Autodesk Inventor part; units mm, degrees
ref_plane "YZ Plane" through (0, 0, 0) normal (1, 0, 0) x (0, 1, 0)
ref_plane "XZ Plane" through (0, 0, 0) normal (0, 1, 0) x (-1, 0, 0)
ref_plane "XY Plane" through (0, 0, 0) normal (0, 0, 1) x (1, 0, 0)
sketch "Sketch4" plane through (0, 0, 0) normal (0, 0, 1) x (1, 0, 0)
  arc A0 (-0.0698, 6.3496) -> (6.1152, -1.7109) centre (0, 0) ccw
  arc A1 (-0.9946, 7.5548) -> (7.04, -2.916) centre (0, 0) ccw
  line L0 (0, 0) -> (0, 7.9375) construction
  line L1 (-0.0698, 6.3496) -> (6.1152, -1.7109) construction
  line L2 (-0.0698, 6.3496) -> (-0.9946, 7.5548)
  line L3 (6.1152, -1.7109) -> (7.04, -2.916)
  circle A2 centre (0, 0) radius 6.35
  dimension "d10" = 12.7
  dimension "d11" = 1.27
  dimension "d12" = 37.5
  dimension "d13" = 10.16
extrude "Extrusion3" add sketch "Sketch4" along normal mid plane 38.1 contours A0 L3 A1 L2
sketch "Sketch5" plane through (0, 0, 0) normal (0, 0, 1) x (1, 0, 0)
  arc A0 (-0.9946, 7.5548) -> (7.04, -2.916) centre (0, 0) ccw
  line L0 (-7.62, 0) -> (-7.62, -29.21)
  line L1 (-7.62, -29.21) -> (0, -29.21)
  line L2 (0, -29.21) -> (0, -7.62)
  circle A1 centre (0, 0) radius 7.9375
  dimension "d16" = 21.59
extrude "Extrusion4" add sketch "Sketch5" along normal mid plane 38.1 contours A0 L2 A1 L0 | A1 L2 L1 L0 picked at (-7.3048, -2.4081)
sketch "Sketch6" plane through (0, -29.21, 19.05) normal (1, 0, 0) x (0, 0, -1)
  line L0 (0, 21.59) -> (38.1, 21.59)
  line L1 (38.1, 21.59) -> (38.1, 0)
  line L2 (0, 0) -> (38.1, 0)
  line L3 (0, 0) -> (0, 21.59)
  line L4 (19.05, 0) -> (19.05, 21.59) construction
  point P0 (19.05, 29.21)
  point P1 (19.05, 5.08)
  dimension "d30" = 5.08
  dimension "d31" = 0
hole "Hole1" at (0, -24.13, 0) direction (-1, 0, 0) diameter 3.5052 end through all countersink diameter 7.112 countersink angle 82
sketch "Sketch10" plane through (-7.62, -29.21, 19.05) normal (0, -1, 0) x (1, 0, 0)
  line L0 (0, -38.1) -> (0, 0)
  line L1 (7.62, -38.1) -> (0, -38.1)
  line L2 (7.62, 0) -> (7.62, -38.1)
  line L3 (0, 0) -> (7.62, 0)
  line L4 (3.81, -38.1) -> (3.81, 0) construction
  spline S0 degree 2 poles (2.8014, -21.2421) (3.1307, -21.2421) (3.7235, -21.4768) (3.9294, -21.6867) knots 0 0 0 1 2 2 2
  spline S1 degree 2 poles (3.9294, -21.6867) (4.1887, -21.9502) (4.4563, -22.6624) (4.4563, -23.2058) knots 0 0 0 1 2 2 2
  line L5 (4.4563, -23.2058) -> (4.4563, -23.778)
  line L6 (4.4563, -23.778) -> (6.35, -23.778)
  line L7 (6.35, -23.778) -> (6.35, -24.4532)
  line L8 (6.35, -24.4532) -> (1.27, -24.4532)
  line L9 (1.27, -24.4532) -> (1.27, -23.177)
  spline S2 degree 2 poles (1.27, -23.177) (1.27, -22.7241) (1.4182, -22.0902) (1.587, -21.8473) knots 0 0 0 1 2 2 2
  spline S3 degree 2 poles (1.587, -21.8473) (1.7805, -21.5632) (2.3774, -21.2421) (2.8014, -21.2421) knots 0 0 0 1 2 2 2
  spline S4 degree 2 poles (2.822, -21.9461) (2.5585, -21.9461) (2.1716, -22.1272) (2.0481, -22.3125) knots 0 0 0 1 2 2 2
  spline S5 degree 2 poles (2.0481, -22.3125) (1.941, -22.473) (1.8546, -22.9012) (1.8546, -23.2182) knots 0 0 0 1 2 2 2
  line L10 (1.8546, -23.2182) -> (1.8546, -23.778)
  line L11 (1.8546, -23.778) -> (3.88, -23.778)
  line L12 (3.88, -23.778) -> (3.88, -23.317)
  spline S6 degree 2 poles (3.88, -23.317) (3.88, -22.9053) (3.7482, -22.3989) (3.5753, -22.2343) knots 0 0 0 1 2 2 2
  spline S7 degree 2 poles (3.5753, -22.2343) (3.423, -22.0819) (3.0649, -21.9461) (2.822, -21.9461) knots 0 0 0 1 2 2 2
  line L13 (1.27, -16.9155) -> (6.35, -18.6651)
  line L14 (6.35, -18.6651) -> (6.35, -19.3937)
  line L15 (6.35, -19.3937) -> (1.27, -21.1433)
  line L16 (1.27, -21.1433) -> (1.27, -20.4188)
  line L17 (1.27, -20.4188) -> (5.4896, -19.0109)
  line L18 (5.4896, -19.0109) -> (1.27, -17.603)
  line L19 (1.27, -17.603) -> (1.27, -16.9155)
  line L20 (6.35, -13.3834) -> (6.35, -16.5162)
  line L21 (6.35, -16.5162) -> (5.6296, -16.5162)
  spline S8 degree 2 poles (5.6296, -16.5162) (5.3126, -16.1786) (4.7239, -15.5776) (4.4069, -15.2894) knots 0 0 0 1 2 2 2
  spline S9 degree 2 poles (4.4069, -15.2894) (3.7688, -14.7089) (3.0031, -14.2849) (2.5956, -14.2849) knots 0 0 0 1 2 2 2
  spline S10 degree 2 poles (2.5956, -14.2849) (2.3815, -14.2849) (2.0604, -14.4167) (1.9575, -14.536) knots 0 0 0 1 2 2 2
  spline S11 degree 2 poles (1.9575, -14.536) (1.8546, -14.6554) (1.7517, -14.9683) (1.7517, -15.1577) knots 0 0 0 1 2 2 2
  spline S12 degree 2 poles (1.7517, -15.1577) (1.7517, -15.3388) (1.8422, -15.7093) (1.9122, -15.8781) knots 0 0 0 1 2 2 2
  spline S13 degree 2 poles (1.9122, -15.8781) (1.9698, -16.0222) (2.1345, -16.2898) (2.1921, -16.3721) knots 0 0 0 1 2 2 2
  line L22 (2.1921, -16.3721) -> (2.1921, -16.4091)
  line L23 (2.1921, -16.4091) -> (1.4676, -16.4091)
  spline S14 degree 2 poles (1.4676, -16.4091) (1.3647, -16.1992) (1.163, -15.4458) (1.163, -15.1083) knots 0 0 0 1 2 2 2
  spline S15 degree 2 poles (1.163, -15.1083) (1.163, -14.3961) (1.9163, -13.5933) (2.5585, -13.5933) knots 0 0 0 1 2 2 2
  spline S16 degree 2 poles (2.5585, -13.5933) (2.859, -13.5933) (3.3613, -13.7333) (3.5753, -13.8568) knots 0 0 0 1 2 2 2
  spline S17 degree 2 poles (3.5753, -13.8568) (3.7976, -13.9803) (4.234, -14.3384) (4.444, -14.536) knots 0 0 0 1 2 2 2
  spline S18 degree 2 poles (4.444, -14.536) (4.7939, -14.8571) (5.5431, -15.6434) (5.7613, -15.8781) knots 0 0 0 1 2 2 2
  line L24 (5.7613, -15.8781) -> (5.7613, -13.3834)
  line L25 (5.7613, -13.3834) -> (6.35, -13.3834)
  point P0 (7.62, -19.05)
extrude "Text" cut sketch "Sketch10" against normal blind 1.143 contours S0 S1 L5 L6 L7 L8 L9 S2 S3 | L13 L14 L15 L16 L17 L18 L19 | L20 L21 S8 S9 S10 S11 S12 S13 L22 L23 S14 S15 S16 S17 S18 L24 L25
equation "\"d10\" = shadeDiameter"
equation "\"d11\" = shadeHolderWallThickness"
equation "\"d13\" = openingForShade"
equation "\"d14\" = partWidth"
equation "\"d16\" = flatBelowShade"
equation "\"d17\" = partWidth"
equation "\"d28\" = textDepth"
equation "\"shadeDiameter\" = 12.7"
equation "\"partWidth\" = 38.1"
equation "\"backThickness\" = 1.905"
equation "\"backHeight\" = 25.4"
equation "\"cutTiltAngle\" = 52.5deg"
equation "\"flatBelowShade\" = 21.59"
equation "\"shadeHolderWallThickness\" = 1.27"
equation "\"openingForShade\" = 10.16"
equation "\"textDepth\" = 1.143"
equation "\"holeHeightAboveBottom\" = 5.08"
properties part number "shadeHolderSideWindow"
Check sheet for the modelled part. Datum: model origin and axes. Units: mm. A direction names the side the tool comes from. Give positions to 0.01 mm unless a question says otherwise; leave off trailing zeros. Loops run counter-clockwise (first coordinate to the right, second up) from the corner with the lowest first, then second, coordinate; pieces in that order, holes last. Notation, with made-up numbers: (32, 19.25) - (37, 19.25) arc R11 cw to (37, 31.25) - close; hole circle Ø8 at (-16, 24.5). An arc over 180 degrees is marked (long way). One line per question, with ' | ' between items. Start each with the question number.
1. Material ranges on line 1 along Y through (x, z) = (-4.5, 1); line 2 along Y through (x, z) = (-5.3, 0); line 3 along X through (y, z) = (-20, 8.5), recorded low to high. Write a range as [from, to].
2. Gauge pin test, flat ends, axial feed: pin 1 Ø0.9 at (y, z) = (-28.5, 4.5) entering from +X; pin 2 Ø4.5 at (y, z) = (-24.13, 0) entering from +X; pin 3 Ø1 at (x, y) = (2.5, -3.5) entering from -Z. Record the tip position at first contact, or that the pin passes through.
3. Cross-section at C-C, the plane x = 5. Enter the section's corners in (y, z), plus the area to 3 significant figures.
4. Cross-section at D-D, the plane y = -17.5. Enter the section's corners in (x, z), plus the area to 3 significant figures.
5. Set-up check for faces 4 (the flat face through (-5, -29.21, -4)), 5 (the flat face through (0, -19, 0)), 6 (the flat face through (-5, -29, -4.728)): record each of +Z, -Z, +X, -X, +Y, -Y from which the full face is reachable in a straight line by a thin tool's end or side.
6. Cross-section at A-A, the plane y = -24.13. Enter the section's corners in (x, z), plus the area to 3 significant figures.
7. Cross-section at B-B, the plane z = 11. Enter the section's corners in (x, y).
8. Draft check along Z on faces 1 (the flat face through (-4, -15, 19.05)), 2 (the flat face through (-4, -29.21, 0)), 3 (the flat face through (-3.846, -28.647, 1.272)). Enter one of: released by +Z, released by -Z, zero draft, split by the parting line, or undercut.
Check result:
1) line 1: y = [-28.07, -25.57], [-22.69, -4.48], [4.48, 6.15] | line 2: y = [-29.21, -25.88], [-22.38, -3.5], [3.5, 5.47] | line 3: x = [-7.62, 0]
2) pin 1: stops at x = 0 | pin 2: stops at x = -1.5 | pin 3: passes through
3) outline: (-5.75, -19.05) - (-3.91, -19.05) - (-3.91, 19.05) - (-5.75, 19.05) - close | area: 69.9 mm2
4) outline: (-7.62, -19.05) - (0, -19.05) - (0, 19.05) - (-7.62, 19.05) - close | area: 290 mm2
5) face 4: +Z, -Z, +X, -X, -Y | face 5: +Z, -Z, +X, -Y | face 6: -Y
6) outline: (-7.62, -19.05) - (0, -19.05) - (0, -3.56) - (-2.07, -1.75) - (-7.62, -1.75) - close; (-7.62, 1.75) - (-2.07, 1.75) - (0, 3.56) - (0, 19.05) - (-7.62, 19.05) - close | area: 260 mm2
7) outline: (-7.62, -29.21) - (0, -29.21) - (0, -7.62) arc R7.62 ccw to (7.04, -2.92) - (6.12, -1.71) arc R6.35 cw (long way) to (-0.07, 6.35) - (-0.99, 7.55) arc R7.62 ccw to (-7.62, 0) - close
8) face 1: released by +Z | face 2: zero draft | face 3: undercut
